```python
from build123d import *

# Parameters (mm, degrees)
RESSALTO_EXTRUS_O1_DEPTH = 5
RESSALTO_EXTRUS_O2_DEPTH = 22.95
ESBO_O3_R                = 1.38
CORTE_EXTRUS_O1_DEPTH    = 5


with BuildPart() as part:
    # Esboço1 → Ressalto-extrusão1 (new body)
    with BuildSketch(Plane.XY):
        with BuildLine():
            Line((-78, -61.175), (78, -61.175))
            ThreePointArc((78, -61.175), (80.5, -58.675), (78, -56.175))
            ThreePointArc((78, -56.175), (75.75493597, -50.75493597), (81.175, -53))
            ThreePointArc((81.175, -53), (83.675, -55.5), (86.175, -53))
            Line((86.175, -53), (86.175, 53))
            ThreePointArc((86.175, 53), (83.675, 55.5), (81.175, 53))
            ThreePointArc((81.175, 53), (75.756150129, 50.753722467), (77.996566768, 56.174998144))
            ThreePointArc((77.996566768, 56.174998144), (80.493861975, 58.677700014), (77.991160104, 61.174995221))
            Line((77.991160104, 61.174995221), (-78, 61.174995221))
            ThreePointArc((-78, 61.174995221), (-80.5, 58.674995221), (-78, 56.174995221))
            ThreePointArc((-78, 56.174995221), (-75.75493597, 50.75493119), (-81.175, 52.999995221))
            ThreePointArc((-81.175, 52.999995221), (-83.675, 55.499995221), (-86.175, 52.999995221))
            Line((-86.175, 52.999995221), (-86.175, -53))
            ThreePointArc((-86.175, -53), (-83.675, -55.5), (-81.175, -53))
            ThreePointArc((-81.175, -53), (-75.75493597, -50.75493597), (-78, -56.175))
            ThreePointArc((-78, -56.175), (-80.5, -58.675), (-78, -61.175))
        make_face()
    extrude(amount=RESSALTO_EXTRUS_O1_DEPTH)

    # Esboço2 → Ressalto-extrusão2 (add)
    with BuildSketch(Plane.XY.offset(5)):
        with BuildLine():
            Line((-78, -56.175), (-35.5, -56.175))
            Line((-35.5, -56.175), (-35.5, -60.212223694))
            Line((-35.5, -60.212223694), (-78, -61.175))
            ThreePointArc((-78, -61.175), (-80.5, -58.675), (-78, -56.175))
        make_face()
        with BuildLine():
            Line((78, -61.175), (65.099265532, -61.175))
            Line((65.099265532, -61.175), (65.099265532, -56.175))
            Line((65.099265532, -56.175), (78, -56.175))
            ThreePointArc((78, -56.175), (80.5, -58.675), (78, -61.175))
        make_face()
    extrude(amount=RESSALTO_EXTRUS_O2_DEPTH)

    # Esboço3 → Corte-extrusão1 (cut)
    with BuildSketch(Plane.XY.offset(5)):
        with Locations((59.125349465, -41.637776306)):
            Circle(ESBO_O3_R)
        with Locations((59.125349465, 16.362223694)):
            Circle(ESBO_O3_R)
        with Locations((-26.874650535, -41.637776306)):
            Circle(ESBO_O3_R)
        with Locations((-26.874650535, 16.362223694)):
            Circle(ESBO_O3_R)
    extrude(amount=-CORTE_EXTRUS_O1_DEPTH, mode=Mode.SUBTRACT)


solid = part.part
```
Read the model definition and answer for the solid it produces. Units are mm, in the model's axes. A direction names the side the tool comes from. Coordinates: 2 decimals unless noted, no trailing zeros. Loops run counter-clockwise (first coordinate to the right, second up) from the corner with the lowest first, then second, coordinate; pieces in that order, holes last.
(1) A tool of negligible diameter and unlimited length cuts with its end or side. For faces 5 (the face through (-35.5, -58, 16)), 6 (the face through (-57, -56.175, 16)), 7 (the face through (-80.5, -58.7, 13.8)), from which of +Z, -Z, +X, -X, +Y, -Y can it reach the whole face along a straight path? Write none if from no direction.
Solution:
face 5: +Z, +Y, -Y
face 6: +Z, +X, -X, +Y
face 7: +Z, -Z, -X
(2) The mould has two halves that part along Y. Classify faces 1 (the face through (75.83, 50.68, 2.46)), 2 (the face through (71, -56.175, 16)), 3 (the face through (17, -61.175, 4.6)), 4 (the face through (75.68, -50.83, 2.46)): released by +Y, released by -Y, zero draft, split by the parting line, or undercut.
Solution:
face 1: undercut
face 2: released by +Y
face 3: released by -Y
face 4: undercut
(3) Consider line 1 along Y through (x, z) = (-78, 2.85) (3 decimals); line 2 along X through (y, z) = (-53, 1.9) (3 decimals); line 3 along Z through (x, y) = (71, 22). Determine where each line is inside the solid, lowest interval first.
Solution:
line 1: y = -61.175 to -56.175, -49.825 to 49.825, 56.175 to 61.175
line 2: x = -86.175 to -81.175, -74.825 to 74.825, 81.175 to 86.175
line 3: z = 0 to 5
(4) The part is cut by section C-C (y = -31). Determine the outline of the cut face in (x, z) (3 decimals).
Solution:
outline: (-86.175, 0) - (86.175, 0) - (86.175, 5) - (-86.175, 5) - close
(5) The part is cut by section D-D (x = -39). Determine the outline of the cut face in (y, z) (3 decimals), and give its area (3 significant figures).
Solution:
outline: (-61.175, 0) - (61.175, 0) - (61.175, 5) - (-56.175, 5) - (-56.175, 27.95) - (-60.292, 27.95) - (-60.292, 5) - (-61.175, 5) - close
area: 706 mm2
(6) The part is cut by section A-A (z = 23.75). Determine the outline of the cut face in (x, y) (3 decimals), and give its area (3 significant figures).
Solution:
outline: (-78, -61.175) - (-35.5, -60.212) - (-35.5, -56.175) - (-78, -56.175) arc R2.5 ccw to start; (65.099, -61.175) - (78, -61.175) arc R2.5 ccw to (78, -56.175) - (65.099, -56.175) - close
area: 276 mm2
(7) Flat-ended cylindrical pins translate along their axes: pin 1 Ø8 at (x, y) = (-43.5, 4) entering from +Z; pin 2 Ø10.5 at (x, z) = (69, 15.5) entering from +Y (3 decimals); pin 3 Ø4.5 at (y, z) = (-58.5, 15.5) entering from +X. Find the tip coordinate at first contact, or state that the pin passes through.
Solution:
pin 1: stops at z = 5
pin 2: stops at y = -56.175
pin 3: stops at x = 80.5
